from build123d import *

# Parameters (mm, degrees)
SKETCH1_R           = 4.1
BOSS_EXTRUDE1_DEPTH = 2
SKETCH2_R           = 1.5
BOSS_EXTRUDE2_DEPTH = 3


with BuildPart() as part:
    # Sketch1 → Boss-Extrude1 (new body)
    with BuildSketch(Plane(origin=(0, 0, 0), x_dir=(1, 0, 0), z_dir=(0, 1, 0))):
        with BuildLine():
            Line((6.880964228, 1.749997239), (31.880964166, 1.749997239))
            ThreePointArc((31.880964166, 1.749997239), (36.598148239, 4.042144166), (37.711172654, 9.167272434))
            ThreePointArc((37.711172654, 9.167272434), (36.026057764, 14.43241452), (33.609947488, 19.40471223))
            ThreePointArc((33.609947488, 19.40471223), (34.250491945, 21.795256686), (36.641036401, 21.15471223))
            ThreePointArc((36.641036401, 21.15471223), (42.309424459, 0), (36.641036401, -21.15471223))
            ThreePointArc((36.641036401, -21.15471223), (34.250491945, -21.795256686), (33.609947488, -19.40471223))
            ThreePointArc((33.609947488, -19.40471223), (36.026056514, -14.432417639), (37.711171067, -9.167278965))
            ThreePointArc((37.711171067, -9.167278965), (36.598147218, -4.042150095), (31.880962823, -1.750002761))
            Line((31.880962823, -1.750002761), (6.880962823, -1.750002761))
            ThreePointArc((6.880962823, -1.750002761), (-0.000729594, -7.100011163), (-6.881322337, -1.748588554))
            Line((-6.881322337, -1.748588554), (-15.881322337, -1.748588554))
            ThreePointArc((-15.881322337, -1.748588554), (-16.588429118, -1.455695335), (-16.881322337, -0.748588554))
            Line((-16.881322337, -0.748588554), (-16.881322337, 0.748588554))
            ThreePointArc((-16.881322337, 0.748588554), (-16.588429118, 1.455695335), (-15.881322337, 1.748588554))
            Line((-15.881322337, 1.748588554), (-6.881322337, 1.748588554))
            ThreePointArc((-6.881322337, 1.748588554), (-0.000726746, 7.100011163), (6.880964228, 1.749997239))
        make_face()
        Circle(SKETCH1_R, mode=Mode.SUBTRACT)
    extrude(amount=BOSS_EXTRUDE1_DEPTH)

    # Sketch2 → Boss-Extrude2 (add)
    with BuildSketch(Plane(origin=(0, 2, 0), x_dir=(1, 0, 0), z_dir=(0, 1, 0))):
        with Locations((36.759322225, 17.141153462)):
            Circle(SKETCH2_R)
        with Locations((40.559424459, 0)):
            Circle(SKETCH2_R)
        with Locations((36.759322225, -17.141153462)):
            Circle(SKETCH2_R)
    extrude(amount=BOSS_EXTRUDE2_DEPTH)


solid = part.part
Verification items for the finished model (mm, model axes). A direction names the side the tool comes from. Round coordinates to 2 decimals unless told otherwise and drop trailing zeros. Order: outer loops, then holes, each group sorted by start corner. A loop starts at its lowest first (then second) coordinate and runs counter-clockwise, first axis right, second up.
1. Section check A-A on y = 1.1. Record the cut outline in (x, z), then the cut area to 3 significant figures.
Final values:
outline: (-16.88, -0.75) arc R1 ccw to (-15.88, -1.75) - (-6.88, -1.75) arc R7.1 ccw to (6.88, -1.75) - (31.88, -1.75) arc R6 cw to (37.71, -9.17) arc R38.81 cw to (33.61, -19.4) arc R1.75 ccw to (36.64, -21.15) arc R42.31 ccw to (36.64, 21.15) arc R1.75 ccw to (33.61, 19.4) arc R38.81 cw to (37.71, 9.17) arc R6 cw to (31.88, 1.75) - (6.88, 1.75) arc R7.1 ccw to (-6.88, 1.75) - (-15.88, 1.75) arc R1 ccw to (-16.88, 0.75) - close; hole circle Ø8.2 at (0, 0)
area: 432 mm2
2. Release check for a two-part mould opening along X. For faces 1 (the cylindrical face through (-0.1, 1, -7.1)), 2 (the cylindrical face through (36, 1, 14.5)), 3 (the cylindrical face through (38.19, 3.48, -17.59)) record: +X half, -X half, draft (parallel to the pull), parting line (faces both ways), or undercut.
Final values:
face 1: undercut
face 2: -X half
face 3: parting line
3. Thickness scan on L1, parallel to Z at x = 0, y = 0.5; L2, parallel to X at y = 1.4, z = 0; L3, parallel to Z at x = 22, y = 1.25. Record the ranges inside material, lowest first.
Final values:
L1: z = -7.1 to -4.1, 4.1 to 7.1
L2: x = -16.88 to -4.1, 4.1 to 42.31
L3: z = -1.75 to 1.75
4. Access from +Z, -Z, +X, -X, +Y, -Y to the whole of each face (thin tool, end or side, straight path). Record for faces 4 (the flat face through (19, 1, -1.75)), 5 (the flat face through (20, 1, 1.75)), 6 (the cylindrical face through (38.19, 3.48, 16.69)), 7 (the flat face through (-11, 1, -1.749)).
Final values:
face 4: -Z, +Y, -Y
face 5: +Z, +Y, -Y
face 6: +Y
face 7: -Z, -X, +Y, -Y
5. Go/stop test with flat-tipped pins: P1, Ø1.6, axis at x = 14.5, y = 1, coming from the +Z side; P2, Ø7.5, axis at x = 0, z = 0, coming from the +Y side; P3, Ø2, axis at x = -13, y = 1, coming from the +Z side; P4, Ø6, axis at x = -10.5, z = 4, coming from the +Y side. Record where each tip stops, or that it passes through.
Final values:
P1: stops at z = 1.75
P2: passes through
P3: stops at z = 1.75
P4: stops at y = 2
6. Section check B-B on x = 0. Record the cut outline in (y, z), then the cut area to 3 significant figures.
Final values:
outline: (0, -7.1) - (2, -7.1) - (2, -4.1) - (0, -4.1) - close; (0, 4.1) - (2, 4.1) - (2, 7.1) - (0, 7.1) - close
area: 12.0 mm2
7. Section check C-C on z = 5. Record the cut outline in (x, y), then the cut area to 3 significant figures.
Final values:
outline: (-5.04, 0) - (5.04, 0) - (5.04, 2) - (-5.04, 2) - close; (37.21, 0) - (42.01, 0) - (42.01, 2) - (37.21, 2) - close
area: 29.8 mm2
8. Section check D-D on x = 24. Record the cut outline in (y, z).
Final values:
outline: (0, -1.75) - (2, -1.75) - (2, 1.75) - (0, 1.75) - close
